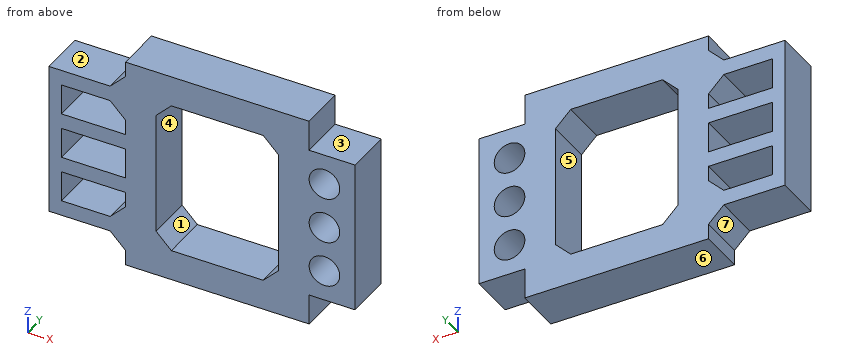
```python
from build123d import *

# Parameters (mm, degrees)
F0_R     = 10
F0_W     = 41.765921
F0_H     = 20
F1_DEPTH = 30


with BuildPart() as f1:
    # F0 (on Front) → F1 (new body)
    with BuildSketch(Plane.XZ):
        Polygon((0, 10), (0, 0), (120, 0), (120, 20), (150, 20), (150, 120), (120, 120), (120, 140), (0, 140), (0, 130), (-10, 120), (-19.487179, 120), (-50, 120), (-50, 20), (-19.487179, 20), (-10, 20), align=None)
        Polygon((-41.765921, 30), (-41.765921, 50), (0, 50), (0, 40), (-10, 30), align=None, mode=Mode.SUBTRACT)
        with Locations((130, 40)):
            Circle(F0_R, mode=Mode.SUBTRACT)
        with Locations((-20.88296, 70)):
            Rectangle(F0_W, F0_H, mode=Mode.SUBTRACT)
        Polygon((-41.765921, 90), (-41.765921, 110), (-10, 110), (0, 100), (0, 90), align=None, mode=Mode.SUBTRACT)
        Polygon((20, 110), (30, 120), (90, 120), (100, 110), (100, 30), (90, 20), (30, 20), (20, 30), align=None, mode=Mode.SUBTRACT)
        with Locations((130, 70)):
            Circle(F0_R, mode=Mode.SUBTRACT)
        with Locations((130, 100)):
            Circle(F0_R, mode=Mode.SUBTRACT)
    extrude(amount=F1_DEPTH)


solid = f1.part
```
Read the model definition and answer for the solid it produces. Units are mm, in the model's axes. Face numbers are marked on the shaded views. A direction names the side the tool comes from. Coordinates: 2 decimals unless noted, no trailing zeros. Write each loop counter-clockwise with the first axis right and the second up, starting at its lowest first coordinate (ties: lowest second). Pieces come first, ordered by that corner, then holes. Notation, with made-up numbers: (-18.5, -18.75) - (8.5, -18.75) arc R24 cw to (8.5, -7.75) - close; hole circle Ø2 at (-20, -15.5). An arc over 180 degrees is marked (long way). Answer as a JSON object with one key per item and string values. Group by question number.
1. A cutting plane is placed at B-B (z = 70). Determine the outline of the cut face in (x, y), plus the area to 3 significant figures.
2. A cutting plane is placed at D-D (z = 27). Determine the outline of the cut face in (x, y).
3. Each of these flat-tipped pins is pushed along its axis until it touches: P1, Ø15, axis at x = -17, y = -13, coming from the +Z side; P2, Ø9, axis at x = 135, y = -18.5, coming from the +Z side; P3, Ø2, axis at y = -21.5, z = 14.5, coming from the +X side; P4, Ø16, axis at x = 130, z = 40, coming from the +Y side. Where does it stop, or does it pass through?
4. The mould has two halves that part along X. Classify the marked faces 4, 5, 6 and 7: +X half, -X half, draft (parallel to the pull), parting line (faces both ways), or undercut.
5. A cutting plane is placed at A-A (x = 130). Determine the outline of the cut face in (y, z).
6. A cutting plane is placed at C-C (x = 35). Determine the outline of the cut face in (y, z), plus the area to 3 significant figures.
7. Which of the six approach directions +Z, -Z, +X, -X, +Y, -Y give full straight-line access (tool end or side, diameter ignored) to the marked faces 1, 2 and 3?
8. Consider L1, parallel to Z at x = 130, y = -18.75; L2, parallel to Z at x = 72.5, y = -12.5; L3, parallel to X at y = -9.25, z = 88. Determine where each line is inside the solid, lowest interval first. Write a range as [from, to].
Worked out:
{
 "1": {"outline": "(-50, -30) - (-41.77, -30) - (-41.77, 0) - (-50, 0) - close; (0, -30) - (20, -30) - (20, 0) - (0, 0) - close; (100, -30) - (120, -30) - (120, 0) - (100, 0) - close; (140, -30) - (150, -30) - (150, 0) - (140, 0) - close", "area": "1,750 mm²"},
 "2": {"outline": "(-50, -30) - (23, -30) - (23, 0) - (-50, 0) - close; (97, -30) - (150, -30) - (150, 0) - (97, 0) - close"},
 "3": {"P1": "stops at z = 120.5", "P2": "stops at z = 120", "P3": "stops at x = 120", "P4": "passes through"},
 "4": {"face 4": "undercut", "face 5": "undercut", "face 6": "draft", "face 7": "-X half"},
 "5": {"outline": "(-30, 20) - (0, 20) - (0, 30) - (-30, 30) - close; (-30, 50) - (0, 50) - (0, 60) - (-30, 60) - close; (-30, 80) - (0, 80) - (0, 90) - (-30, 90) - close; (-30, 110) - (0, 110) - (0, 120) - (-30, 120) - close"},
 "6": {"outline": "(-30, 0) - (0, 0) - (0, 20) - (-30, 20) - close; (-30, 120) - (0, 120) - (0, 140) - (-30, 140) - close", "area": "1,200 mm²"},
 "7": {"face 1": "+Y, -Y", "face 2": "+Z, -X, +Y, -Y", "face 3": "+Z, +X, +Y, -Y"},
 "8": {"L1": "z = [20, 30], [50, 60], [80, 90], [110, 120]", "L2": "z = [0, 20], [120, 140]", "L3": "x = [-50, 20], [100, 150]"}
}
